The listing builds one solid part. Answer for the finished solid, in the listing's coordinates (mm). A direction names the side the tool comes from. Coordinates: 2 decimals unless noted, no trailing zeros. Loops run counter-clockwise (first coordinate to the right, second up) from the corner with the lowest first, then second, coordinate; pieces in that order, holes last. Notation, with made-up numbers: M 48.5,-13.5 L 100.5,-13.5 A19 ccw 100.5,18.5 Z; hole C 3.5,33 d7. An arc over 180 degrees is marked long. Return JSON: item names as keys, results as strings. Group by question number.
1. Straight lines are drawn through the part: L1, parallel to X at y = -0.05, z = 0.75; L2, parallel to X at y = 0.35, z = -1; L3, parallel to Z at x = -35.5, y = 1.6. For each, find the intervals that lie inside material, in ascending order. Write a range as from..to.
2. Section C-C (x = -39) is taken. Write down the section's boundary in (y, z), then the cut area to 3 significant figures.
3. Section A-A (y = 0) is taken. Write down the section's boundary in (x, z), then the cut area to 3 significant figures.
4. Section B-B (z = 1.15) is taken. Write down the section's boundary in (x, y), then the cut area to 3 significant figures.
5. Given P1, Ø1, axis at x = -33.5, z = 1, coming from the +Y side; P2, Ø1.6, axis at x = -18.5, z = 1, coming from the -Y side; P3, Ø0.6, axis at x = -29.5, y = 1, coming from the +Z side; P4, Ø1, axis at x = -20.5, y = 1.5, coming from the +Z side, each flat-ended and moving along its own axis, determine where each tip first touches the part or whether it passes through.
6. Which of the six approach directions +Z, -Z, +X, -X, +Y, -Y give full straight-line access (tool end or side, diameter ignored) to faces 1 (the face through (-26, 1, 0)), 2 (the face through (-26, -0.819, 1)), 3 (the face through (-27, 2, -1))?
7. The mould has two halves that part along Y. Classify faces 4 (the face through (-26, -1, 0)), 5 (the face through (-27, 0.819, 1)), 6 (the face through (-45.103, 0.246, 0.028)): pulls with the +Y half, pulls with the -Y half, needs draft (parallel to the pull), parting line crosses it, or undercut.
8. Section D-D (y = -1.55) is taken. Write down the section's boundary in (x, z).
```python
from build123d import *

# Parameters (mm, degrees)
SKETCH_1_R      = 0.819112032
EXTRUDE_1_DEPTH = 2
EXTRUDE_START   = 2
SKETCH_2_R      = 0.819112032
EXTRUDE_2_DEPTH = 2


with BuildPart() as part:
    # 草图1 → 凸台-拉伸1 (new body)
    with BuildSketch(Plane.XY):
        with BuildLine():
            Line((-45.884505443, 2), (-7.384505443, 2))
            ThreePointArc((-7.384505443, 2), (-5.384505443, 0), (-7.384505443, -2))
            Line((-7.384505443, -2), (-45.884505443, -2))
            ThreePointArc((-45.884505443, -2), (-47.884505443, 0), (-45.884505443, 2))
        make_face()
        with Locations((-45.884505443, 0)):
            Circle(SKETCH_1_R, mode=Mode.SUBTRACT)
        with Locations((-7.384505443, 0)):
            Circle(SKETCH_1_R, mode=Mode.SUBTRACT)
    extrude(amount=-EXTRUDE_1_DEPTH)

    # 草图2 → 凸台-拉伸2 (add)
    with BuildSketch(Plane.XY.offset(EXTRUDE_START)):
        with BuildLine():
            Line((-44.059935499, 0.819112032), (-9.209075386, 0.819112032))
            ThreePointArc((-9.209075386, 0.819112032), (-5.384505443, 0), (-9.209075386, -0.819112032))
            Line((-9.209075386, -0.819112032), (-44.059935499, -0.819112032))
            ThreePointArc((-44.059935499, -0.819112032), (-47.884505443, 0), (-44.059935499, 0.819112032))
        make_face()
        with Locations((-45.884505443, 0)):
            Circle(SKETCH_2_R, mode=Mode.SUBTRACT)
        with Locations((-7.384505443, 0)):
            Circle(SKETCH_2_R, mode=Mode.SUBTRACT)
    extrude(amount=-EXTRUDE_2_DEPTH)


solid = part.part
```
Worked out:
{
 "1": {"L1": "-47.88..-46.7, -45.07..-8.2, -6.57..-5.39", "L2": "-47.85..-46.63, -45.14..-8.13, -6.64..-5.42", "L3": "-2..0"},
 "2": {"outline": "M -2,-2 L 2,-2 L 2,0 L 0.82,0 L 0.82,2 L -0.82,2 L -0.82,0 L -2,0 Z", "area": "11.3 mm^2"},
 "3": {"outline": "M -47.88,-2 L -46.7,-2 L -46.7,2 L -47.88,2 Z; M -45.07,-2 L -8.2,-2 L -8.2,2 L -45.07,2 Z; M -6.57,-2 L -5.38,-2 L -5.38,2 L -6.57,2 Z", "area": "157 mm^2"},
 "4": {"outline": "M -44.06,-0.82 L -9.21,-0.82 A2 ccw long -9.21,0.82 L -44.06,0.82 A2 ccw long Z; hole C -45.88,0 d1.64; hole C -7.38,0 d1.64", "area": "77.6 mm^2"},
 "5": {"P1": "y = 0.82", "P2": "y = -0.82", "P3": "z = 2", "P4": "z = 0"},
 "6": {"face 1": "+Z, +Y", "face 2": "+Z, -Y", "face 3": "+Z, -Z, +X, -X, +Y"},
 "7": {"face 4": "needs draft", "face 5": "pulls with the +Y half", "face 6": "undercut"},
 "8": {"outline": "M -47.15,-2 L -6.12,-2 L -6.12,2 L -8.65,2 L -8.65,0 L -44.62,0 L -44.62,2 L -47.15,2 Z"}
}
